from build123d import *

# Parameters (mm, degrees)
SKETCH1_W           = 12.7
SKETCH1_H           = 6.35
SKETCH1_W_2         = 38.1
SKETCH1_H_2         = 34.925
BOSS_EXTRUDE1_DEPTH = 6.35
SKETCH2_W           = 4.7625
SKETCH2_H           = 14.2875
SKETCH2_W_2         = 9.525
SKETCH2_H_2         = 3.175
CUT_EXTRUDE1_DEPTH  = 6.35


with BuildPart() as part:
    # Sketch1 → Boss-Extrude1 (new body)
    with BuildSketch(Plane(origin=(0, 0, 0), x_dir=(0, 0, -1), z_dir=(1, 0, 0))):
        Polygon((12.7, 38.1), (12.7, 44.45), (0, 44.45), (0, 0), (6.35, 0), (6.35, 6.35), (19.05, 6.35), (19.05, 0), (31.75, 0), (31.75, 6.35), (38.1, 6.35), (38.1, 0), (44.45, 0), (44.45, 38.1), (38.1, 38.1), (38.1, 44.45), (25.4, 44.45), (25.4, 38.1), align=None)
        Polygon((88.9, 0), (44.45, 38.1), (44.45, 0), (50.8, 0), align=None)
        with Locations((57.15, -38.1)):
            Rectangle(SKETCH1_W, SKETCH1_H)
        with Locations((69.85, -17.4625)):
            Rectangle(SKETCH1_W_2, SKETCH1_H_2)
        with Locations((82.55, -38.1)):
            Rectangle(SKETCH1_W, SKETCH1_H)
    extrude(amount=BOSS_EXTRUDE1_DEPTH)

    # Sketch2 → Cut-Extrude1 (cut)
    with BuildSketch(Plane(origin=(6.35, 0, 0), x_dir=(0, 0, -1), z_dir=(1, 0, 0))):
        with Locations((12.7, 13.49375)):
            Rectangle(SKETCH2_W, SKETCH2_H)
        with Locations((12.7, 15.875)):
            Rectangle(SKETCH2_W_2, SKETCH2_H_2)
        with Locations((19.05, 30.95625)):
            Rectangle(SKETCH2_W, SKETCH2_H)
        with Locations((19.05, 28.575)):
            Rectangle(SKETCH2_W_2, SKETCH2_H_2)
        with Locations((69.85, -27.78125)):
            Rectangle(SKETCH2_W, SKETCH2_H)
        with Locations((69.85, -25.4)):
            Rectangle(SKETCH2_W_2, SKETCH2_H_2)
    extrude(amount=-CUT_EXTRUDE1_DEPTH, mode=Mode.SUBTRACT)


solid = part.part
Design review of the part built by this model. Coordinates are the model's own, in mm. A direction names the side the tool comes from. Round coordinates to 2 decimals unless told otherwise and drop trailing zeros. Order: outer loops, then holes, each group sorted by start corner. A loop starts at its lowest first (then second) coordinate and runs counter-clockwise, first axis right, second up. Notation, with made-up numbers: M 81,83.5 L 99,83.5 A25 ccw 99,115.5 Z; hole C -10,-21.75 d11. An arc over 180 degrees is marked long. Answer as CSV lines item,"result". Start each with the question number.
1) Tool access review of faces 1 (the face through (3, 38.1, -15)), 2 (the face through (3, 19, -15.081)), 3 (the face through (3, -23.812, -66)): name each direction out of +Z, -Z, +X, -X, +Y, -Y from which nothing blocks a thin tool from reaching the whole face with its end or side.
2) Add section D-D (y = 11). Give the boundary of the cut face in (x, z), then the cut area to 3 significant figures.
3) Add section B-B (y = 2). Give the boundary of the cut face in (x, z).
4) Wall thickness on line 1 along Z through (x, y) = (6.25, -29.5); line 2 along Z through (x, y) = (5.75, 38.5); line 3 along Y through (x, z) = (3.75, -23): over which ranges is each line inside the solid? List them lowest first. Write a range as [from, to].
5) For pin 1 Ø1 at (x, y) = (4, 16.5) entering from +Z; pin 2 Ø1 at (x, z) = (4.5, -15.5) entering from +Y; pin 3 Ø0.7 at (x, z) = (4, -9.5) entering from -Y; pin 4 Ø1.2 at (x, z) = (4.5, -17.5) entering from -Y, all flat-tipped, find the tip position at first contact; note any pin that passes through.
6) Add section C-C (z = -41). Give the boundary of the cut face in (x, y), then the cut area to 3 significant figures.
7) The part is to be moulded in two halves that separate along Z. For faces 4 (the face through (3, -26.987, -73)), 5 (the face through (3, -41.275, -57)), 6 (the face through (3, 30.162, -23)), 7 (the face through (3.13, 18.78, -66.99)), say which applies: +Z half, -Z half, draft (parallel to the pull), parting line (faces both ways), or undercut.
8) Add section A-A (y = -29). Give the boundary of the cut face in (x, z), then the cut area to 3 significant figures.
Resolved:
1,face 1,"+X, -X, +Y"
1,face 2,"+X, -X, -Y"
1,face 3,"+X, -X"
2,outline,"M 0,-76.07 L 6.35,-76.07 L 6.35,-15.08 L 0,-15.08 Z; M 0,-10.32 L 6.35,-10.32 L 6.35,0 L 0,0 Z"
2,area,"453 mm^2"
3,outline,"M 0,-86.57 L 6.35,-86.57 L 6.35,-38.1 L 0,-38.1 Z; M 0,-31.75 L 6.35,-31.75 L 6.35,-19.05 L 0,-19.05 Z; M 0,-6.35 L 6.35,-6.35 L 6.35,0 L 0,0 Z"
4,line 1,"[-88.9, -72.23], [-67.47, -50.8]"
4,line 2,"[-38.1, -25.4], [-12.7, 0]"
4,line 3,"[0, 26.99], [30.16, 38.1]"
5,pin 1,"z = 0"
5,pin 2,"y = 38.1"
5,pin 3,"y = 6.35"
5,pin 4,"y = 6.35"
6,outline,"M 0,0 L 6.35,0 L 6.35,38.1 L 0,38.1 Z"
6,area,"242 mm^2"
7,face 4,"undercut"
7,face 5,"draft"
7,face 6,"undercut"
7,face 7,"-Z half"
8,outline,"M 0,-88.9 L 6.35,-88.9 L 6.35,-72.23 L 0,-72.23 Z; M 0,-67.47 L 6.35,-67.47 L 6.35,-50.8 L 0,-50.8 Z"
8,area,"212 mm^2"
